```python
from build123d import *

# Parameters (mm, degrees)
SKETCH1_W           = 80
SKETCH1_H           = 55
BOSS_EXTRUDE1_DEPTH = 10
SKETCH2_W           = 10
SKETCH2_H           = 55
BOSS_EXTRUDE2_DEPTH = 30
SKETCH3_R           = 2
CUT_EXTRUDE1_DEPTH  = 81
SKETCH4_R           = 2.5
CUT_EXTRUDE2_DEPTH  = 30
SKETCH5_R           = 7.5
SKETCH5_R_2         = 2.5
BOSS_EXTRUDE3_DEPTH = 20
SKETCH6_W           = 20.5
SKETCH6_H           = 3.25
CUT_EXTRUDE3_DEPTH  = 5
CUT_EXTRUDE4_DEPTH  = 81


with BuildPart() as part:
    # Sketch1 → Boss-Extrude1 (new body)
    with BuildSketch(Plane(origin=(0, 0, 0), x_dir=(1, 0, 0), z_dir=(0, 1, 0))):
        Rectangle(SKETCH1_W, SKETCH1_H)
    extrude(amount=BOSS_EXTRUDE1_DEPTH)

    # Sketch2 → Boss-Extrude2 (add)
    with BuildSketch(Plane(origin=(0, 10, 0), x_dir=(1, 0, 0), z_dir=(0, 1, 0))):
        with Locations((-35, 0)):
            Rectangle(SKETCH2_W, SKETCH2_H)
        with Locations((35, 0)):
            Rectangle(SKETCH2_W, SKETCH2_H)
    extrude(amount=BOSS_EXTRUDE2_DEPTH)

    # Sketch3 → Cut-Extrude1 (cut, through all)
    with BuildSketch(Plane.ZY.offset(40)):
        with Locations((-23.624192801, 20)):
            Circle(SKETCH3_R)
        with Locations((0.375807199, 20)):
            Circle(SKETCH3_R)
        with Locations((24.375807199, 20)):
            Circle(SKETCH3_R)
        with Locations((-11.624192801, 32)):
            Circle(SKETCH3_R)
        with Locations((12.375807199, 32)):
            Circle(SKETCH3_R)
    extrude(amount=-CUT_EXTRUDE1_DEPTH, mode=Mode.SUBTRACT)

    # Sketch4 → Cut-Extrude2 (cut)
    with BuildSketch(Plane.XZ):
        with Locations((0, 15)):
            Circle(SKETCH4_R)
        with Locations((0, -15)):
            Circle(SKETCH4_R)
    extrude(amount=-CUT_EXTRUDE2_DEPTH, mode=Mode.SUBTRACT)

    # Sketch5 → Boss-Extrude3 (add)
    with BuildSketch(Plane(origin=(0, 10, 0), x_dir=(1, 0, 0), z_dir=(0, 1, 0))):
        with Locations((0, 15)):
            Circle(SKETCH5_R)
        with Locations((0, 15)):
            Circle(SKETCH5_R_2, mode=Mode.SUBTRACT)
        with Locations((0, -15)):
            Circle(SKETCH5_R)
        with Locations((0, -15)):
            Circle(SKETCH5_R_2, mode=Mode.SUBTRACT)
    extrude(amount=BOSS_EXTRUDE3_DEPTH)

    # Sketch6 → Cut-Extrude3 (cut)
    with BuildSketch(Plane.XZ):
        with Locations((0, 9.125)):
            Rectangle(SKETCH6_W, SKETCH6_H)
        with Locations((0, -9.125)):
            Rectangle(SKETCH6_W, SKETCH6_H)
    extrude(amount=-CUT_EXTRUDE3_DEPTH, mode=Mode.SUBTRACT)

    # Sketch7 → Cut-Extrude4 (cut, through all)
    with BuildSketch(Plane(origin=(40, 0, 0), x_dir=(0, 0, -1), z_dir=(1, 0, 0))):
        Polygon((-27.5, 28), (-15.5, 40), (-27.5, 40), align=None)
        Polygon((15.5, 40), (27.5, 28), (27.5, 40), align=None)
    extrude(amount=-CUT_EXTRUDE4_DEPTH, mode=Mode.SUBTRACT)


solid = part.part
```
Check sheet for the modelled part. Datum: model origin and axes. Units: mm. A direction names the side the tool comes from. Give positions to 0.01 mm unless a question says otherwise; leave off trailing zeros. Order: outer loops, then holes, each group sorted by start corner. A loop starts at its lowest first (then second) coordinate and runs counter-clockwise, first axis right, second up. Notation, with made-up numbers: (0.25, 70.5) -> (23.25, 70.5) arc R16 ccw to (23.25, 83.5) -> close; hole circle Ø11 at (58.5, -24). An arc over 180 degrees is marked (long way). Use CSV: the item, a comma, the result in double quotes. Start each with the question number.
1) Sectioned sample at B-B, the plane x = 0. Record the boundary of the cut face in (y, z).
2) Sectioned sample at C-C, the plane z = 9. Record the boundary of the cut face in (x, y).
3) Sectioned sample at D-D, the plane y = 3.5. Record the boundary of the cut face in (x, z).
4) Sectioned sample at A-A, the plane y = 13.5. Record the boundary of the cut face in (x, z), plus the area to 3 significant figures.
5) Mould release check, pull along Z, two halves, no side actions. Record for faces 6 (the face through (0, 2, -10.75)), 7 (the face through (-40, 15, 0)), 8 (the face through (-1, 8, -27.5)): released by +Z, released by -Z, zero draft, split by the parting line, or undercut.
6) Set-up check for faces 1 (the face through (-30, 25, 0)), 2 (the face through (-35.07, 21.35, -25.1)), 3 (the face through (10.25, 2, -9)), 4 (the face through (-1, 0, 0)), 5 (the face through (-1.63, 19.86, 22.32)): record each of +Z, -Z, +X, -X, +Y, -Y from which the full face is reachable in a straight line by a thin tool's end or side.
7) Material ranges on line 1 (Z direction, x = 0, y = 8); line 2 (X direction, y = 13, z = 21.5); line 3 (X direction, y = 36.5, z = -0.5), recorded low to high. Write a range as from..to.
8) Go/stop test with flat-tipped pins: P1, Ø2.5, axis at y = 20, z = 24.38, coming from the -X side; P2, Ø16.5, axis at x = -0.5, z = -16, coming from the +Y side; P3, Ø4, axis at x = 9, z = -10, coming from the -Y side; P4, Ø16.5, axis at x = 15, z = 5.5, coming from the +Y side. Record where each tip stops, or that it passes through.
Recorded:
1,outline,"(0, -27.5) -> (10, -27.5) -> (10, -22.5) -> (30, -22.5) -> (30, -17.5) -> (0, -17.5) -> close; (0, -12.5) -> (30, -12.5) -> (30, -7.5) -> (10, -7.5) -> (10, 7.5) -> (30, 7.5) -> (30, 12.5) -> (0, 12.5) -> (0, 10.75) -> (5, 10.75) -> (5, 7.5) -> (0, 7.5) -> (0, -7.5) -> (5, -7.5) -> (5, -10.75) -> (0, -10.75) -> close; (0, 17.5) -> (30, 17.5) -> (30, 22.5) -> (10, 22.5) -> (10, 27.5) -> (0, 27.5) -> close"
2,outline,"(-40, 0) -> (-10.25, 0) -> (-10.25, 5) -> (10.25, 5) -> (10.25, 0) -> (40, 0) -> (40, 40) -> (30, 40) -> (30, 10) -> (4.5, 10) -> (4.5, 30) -> (-4.5, 30) -> (-4.5, 10) -> (-30, 10) -> (-30, 40) -> (-40, 40) -> close"
3,outline,"(-40, -27.5) -> (40, -27.5) -> (40, 27.5) -> (-40, 27.5) -> close; hole (-10.25, -10.75) -> (10.25, -10.75) -> (10.25, -7.5) -> (-10.25, -7.5) -> close; hole (-10.25, 7.5) -> (10.25, 7.5) -> (10.25, 10.75) -> (-10.25, 10.75) -> close; hole circle Ø5 at (0, -15); hole circle Ø5 at (0, 15)"
4,outline,"(-40, -27.5) -> (-30, -27.5) -> (-30, 27.5) -> (-40, 27.5) -> close; circle Ø15 at (0, -15); circle Ø15 at (0, 15); (30, -27.5) -> (40, -27.5) -> (40, 27.5) -> (30, 27.5) -> close; hole circle Ø5 at (0, -15); hole circle Ø5 at (0, 15)"
4,area,"1,410 mm2"
5,face 6,"undercut"
5,face 7,"zero draft"
5,face 8,"released by -Z"
6,face 1,"+Z, -Z, +Y"
6,face 2,"-X"
6,face 3,"-Y"
6,face 4,"+Z, -Z, +X, -X, -Y"
6,face 5,"+Y"
7,line 1,"-27.5..-17.5, -12.5..12.5, 17.5..27.5"
7,line 2,"-40..-30, -3.74..3.74, 30..40"
7,line 3,"-40..-30, 30..40"
8,P1,"through"
8,P2,"y = 30"
8,P3,"y = 0"
8,P4,"y = 10"
